Work out the finished part from the listing and answer in its coordinate system (mm). A direction names the side the tool comes from. Round coordinates to 2 decimals unless told otherwise and drop trailing zeros. Loops run counter-clockwise (first coordinate to the right, second up) from the corner with the lowest first, then second, coordinate; pieces in that order, holes last.
```python
from build123d import *

# Parameters (mm, degrees)
F1_DEPTH = 2
F2_DEPTH = 8
F3_SIZE  = 1.5


with BuildPart() as f1:
    # F0 (on Top) → F1 (new body)
    with BuildSketch(Plane.XY):
        with BuildLine():
            Line((-3.5, -23.3402318112), (-3.5, -10.0054984883))
            ThreePointArc((-3.5, -10.0054984883), (-8.6446515257, -6.1343296292), (-10.6, 0))
            Line((-10.6, 0), (-10.6, -23.3402318112))
            Line((-10.6, -23.3402318112), (-3.5, -23.3402318112))
        make_face()
        with BuildLine():
            ThreePointArc((10.6, 0), (8.6446515257, -6.1343296292), (3.5, -10.0054984883))
            Line((3.5, -10.0054984883), (3.5, -23.3402318112))
            Line((3.5, -23.3402318112), (10.6, -23.3402318112))
            Line((10.6, -23.3402318112), (10.6, 0))
        make_face()
        with BuildLine():
            Line((3.5, -23.3402318112), (3.5, -10.0054984883))
            ThreePointArc((3.5, -10.0054984883), (2.2665754234, -10.3548363507), (1, -10.5527247666))
            Line((1, -10.5527247666), (1, -23.3402318112))
            Line((1, -23.3402318112), (3.5, -23.3402318112))
        make_face()
        with BuildLine():
            ThreePointArc((-1, -10.5527247666), (-2.2665754234, -10.3548363507), (-3.5, -10.0054984883))
            Line((-3.5, -10.0054984883), (-3.5, -23.3402318112))
            Line((-3.5, -23.3402318112), (-1, -23.3402318112))
            Line((-1, -23.3402318112), (-1, -10.5527247666))
        make_face()
        with BuildLine():
            ThreePointArc((-1, -5.5099909256), (-2.3208923272, -5.0964162708), (-3.5, -4.3714985989))
            Line((-3.5, -4.3714985989), (-3.5, -10.0054984883))
            ThreePointArc((-3.5, -10.0054984883), (-2.2665754234, -10.3548363507), (-1, -10.5527247666))
            Line((-1, -10.5527247666), (-1, -5.5099909256))
        make_face()
        with BuildLine():
            Line((-3.5, -10.0054984883), (-3.5, -4.3714985989))
            ThreePointArc((-3.5, -4.3714985989), (-2.4248711306, 5.0477717856), (5.6, 0))
            ThreePointArc((5.6, 0), (5.0477717856, -2.4248711306), (3.5, -4.3714985989))
            Line((3.5, -4.3714985989), (3.5, -10.0054984883))
            ThreePointArc((3.5, -10.0054984883), (8.6446515257, -6.1343296292), (10.6, 0))
            ThreePointArc((10.6, 0), (0, 10.6), (-10.6, 0))
            ThreePointArc((-10.6, 0), (-8.6446515257, -6.1343296292), (-3.5, -10.0054984883))
        make_face()
        with BuildLine():
            ThreePointArc((-3.5, -1.9364916731), (-1, 3.8729833462), (4, 0))
            ThreePointArc((4, 0), (3.8729833462, -1), (3.5, -1.9364916731))
            Line((3.5, -1.9364916731), (3.5, -4.3714985989))
            ThreePointArc((3.5, -4.3714985989), (5.0477717856, -2.4248711306), (5.6, 0))
            ThreePointArc((5.6, 0), (-2.4248711306, 5.0477717856), (-3.5, -4.3714985989))
            Line((-3.5, -4.3714985989), (-3.5, -1.9364916731))
        make_face()
        with BuildLine():
            Line((3.5, -10.0054984883), (3.5, -4.3714985989))
            ThreePointArc((3.5, -4.3714985989), (2.3208923272, -5.0964162708), (1, -5.5099909256))
            Line((1, -5.5099909256), (1, -10.5527247666))
            ThreePointArc((1, -10.5527247666), (2.2665754234, -10.3548363507), (3.5, -10.0054984883))
        make_face()
        with BuildLine():
            Line((3.5, -4.3714985989), (3.5, -1.9364916731))
            ThreePointArc((3.5, -1.9364916731), (2.4494897428, -3.1622776602), (1, -3.8729833462))
            Line((1, -3.8729833462), (1, -5.5099909256))
            ThreePointArc((1, -5.5099909256), (2.3208923272, -5.0964162708), (3.5, -4.3714985989))
        make_face()
        with BuildLine():
            ThreePointArc((-1, -3.8729833462), (-2.4494897428, -3.1622776602), (-3.5, -1.9364916731))
            Line((-3.5, -1.9364916731), (-3.5, -4.3714985989))
            ThreePointArc((-3.5, -4.3714985989), (-2.3208923272, -5.0964162708), (-1, -5.5099909256))
            Line((-1, -5.5099909256), (-1, -3.8729833462))
        make_face()
    extrude(amount=F1_DEPTH)

    # F0 (on Top) → F2 (join)
    with BuildSketch(Plane.XY):
        with BuildLine():
            ThreePointArc((-3.5, -1.9364916731), (-1, 3.8729833462), (4, 0))
            ThreePointArc((4, 0), (3.8729833462, -1), (3.5, -1.9364916731))
            Line((3.5, -1.9364916731), (3.5, -4.3714985989))
            ThreePointArc((3.5, -4.3714985989), (5.0477717856, -2.4248711306), (5.6, 0))
            ThreePointArc((5.6, 0), (-2.4248711306, 5.0477717856), (-3.5, -4.3714985989))
            Line((-3.5, -4.3714985989), (-3.5, -1.9364916731))
        make_face()
        with BuildLine():
            ThreePointArc((-1, -5.5099909256), (-2.3208923272, -5.0964162708), (-3.5, -4.3714985989))
            Line((-3.5, -4.3714985989), (-3.5, -10.0054984883))
            ThreePointArc((-3.5, -10.0054984883), (-2.2665754234, -10.3548363507), (-1, -10.5527247666))
            Line((-1, -10.5527247666), (-1, -5.5099909256))
        make_face()
        with BuildLine():
            ThreePointArc((-1, -10.5527247666), (-2.2665754234, -10.3548363507), (-3.5, -10.0054984883))
            Line((-3.5, -10.0054984883), (-3.5, -23.3402318112))
            Line((-3.5, -23.3402318112), (-1, -23.3402318112))
            Line((-1, -23.3402318112), (-1, -10.5527247666))
        make_face()
        with BuildLine():
            Line((3.5, -23.3402318112), (3.5, -10.0054984883))
            ThreePointArc((3.5, -10.0054984883), (2.2665754234, -10.3548363507), (1, -10.5527247666))
            Line((1, -10.5527247666), (1, -23.3402318112))
            Line((1, -23.3402318112), (3.5, -23.3402318112))
        make_face()
        with BuildLine():
            Line((3.5, -10.0054984883), (3.5, -4.3714985989))
            ThreePointArc((3.5, -4.3714985989), (2.3208923272, -5.0964162708), (1, -5.5099909256))
            Line((1, -5.5099909256), (1, -10.5527247666))
            ThreePointArc((1, -10.5527247666), (2.2665754234, -10.3548363507), (3.5, -10.0054984883))
        make_face()
        with BuildLine():
            Line((3.5, -4.3714985989), (3.5, -1.9364916731))
            ThreePointArc((3.5, -1.9364916731), (2.4494897428, -3.1622776602), (1, -3.8729833462))
            Line((1, -3.8729833462), (1, -5.5099909256))
            ThreePointArc((1, -5.5099909256), (2.3208923272, -5.0964162708), (3.5, -4.3714985989))
        make_face()
        with BuildLine():
            ThreePointArc((-1, -3.8729833462), (-2.4494897428, -3.1622776602), (-3.5, -1.9364916731))
            Line((-3.5, -1.9364916731), (-3.5, -4.3714985989))
            ThreePointArc((-3.5, -4.3714985989), (-2.3208923272, -5.0964162708), (-1, -5.5099909256))
            Line((-1, -5.5099909256), (-1, -3.8729833462))
        make_face()
    extrude(amount=F2_DEPTH)

    # F3
    f3_edges = [f1.edges().sort_by_distance(p)[0] for p in [
        (0, 10.6, 0),
        (-10.6, -11.670116, 0),
        (-5.8, -23.340232, 0),
        (-1, -13.606608, 0),
        (0, 4, 0),
        (1, -13.606608, 0),
        (5.8, -23.340232, 0),
        (10.6, -11.670116, 0),
    ]]
    chamfer(f3_edges, length=F3_SIZE)


solid = f1.part
```
1. Consider probe 1 along X at (y, z) = (0, 3.75); probe 2 along X at (y, z) = (-5, 7); probe 3 along Y at (x, z) = (0, 5.75). Determine where each line is inside the solid, lowest interval first.
Answer key:
probe 1: x = -5.6 to -4, 4 to 5.6
probe 2: x = -3.5 to -1, 1 to 3.5
probe 3: y = 4 to 5.6
2. Find section A-A (y = -6). Write down the section's boundary in (x, z).
Answer key:
outline: (-10.6, 1.5) - (-9.1, 0) - (-2.5, 0) - (-1, 1.5) - (-1, 8) - (-3.5, 8) - (-3.5, 2) - (-10.6, 2) - close; (1, 1.5) - (2.5, 0) - (9.1, 0) - (10.6, 1.5) - (10.6, 2) - (3.5, 2) - (3.5, 8) - (1, 8) - close
3. Find section B-B (z = 2.5). Write down the section's boundary in (x, y), then the cut area to 3 significant figures.
Answer key:
outline: (-3.5, -23.34) - (-1, -23.34) - (-1, -3.87) arc R4 cw (long way) to (1, -3.87) - (1, -23.34) - (3.5, -23.34) - (3.5, -4.37) arc R5.6 ccw (long way) to (-3.5, -4.37) - close
area: 136 mm2
4. Given pin 1 (3 mm diameter, centred on y = -12.5, z = 4.5, fed in from -X); pin 2 (2 mm diameter, centred on x = 6.5, y = -9, fed in from +Z); pin 3 (9 mm diameter, centred on x = 0, y = 0, fed in from -Z), each flat-ended and moving along its own axis, determine where each tip first touches the part or whether it passes through.
Answer key:
pin 1: stops at x = -3.5
pin 2: stops at z = 2
pin 3: stops at z = 1
5. Determine the mould class of faces 6 (the face through (-9.8, -11.5, 0.7)), 7 (the face through (-1, -14, 5)), 8 (the face through (3, -23.34, 4)) for opening direction X: +X half, -X half, draft (parallel to the pull), parting line (faces both ways), or undercut.
Answer key:
face 6: -X half
face 7: undercut
face 8: draft
6. Find section C-C (x = 0). Write down the section's boundary in (y, z).
Answer key:
outline: (4, 1.5) - (5.5, 0) - (9.1, 0) - (10.6, 1.5) - (10.6, 2) - (5.6, 2) - (5.6, 8) - (4, 8) - close
7. Which of the six approach directions +Z, -Z, +X, -X, +Y, -Y give full straight-line access (tool end or side, diameter ignored) to faces 1 (the face through (-1.8, -13.7, 0.7)), 2 (the face through (1, -13, 5)), 3 (the face through (-3.5, -14, 5)), 4 (the face through (-5, -6, 2)), 5 (the face through (3.5, -14, 5))?
Answer key:
face 1: -Z, -Y
face 2: +Z, -Z, -Y
face 3: +Z, -X, -Y
face 4: +Z
face 5: +Z, +X, -Y
